The figure shows three views and two pictorial views of one solid part (mm, origin at its lowest corner). Answer the questions. Give positions to 0.01 mm unless a question says otherwise; leave off trailing zeros. Loops run counter-clockwise (first coordinate to the right, second up) from the corner with the lowest first, then second, coordinate; pieces in that order, holes last. Notation, with made-up numbers: (88, 69) - (128, 69) arc R22 cw to (128, 86) - close; hole circle Ø4 at (16.25, 87.5). An arc over 180 degrees is marked (long way). Write each question's results on one line, items separated by ' | '.
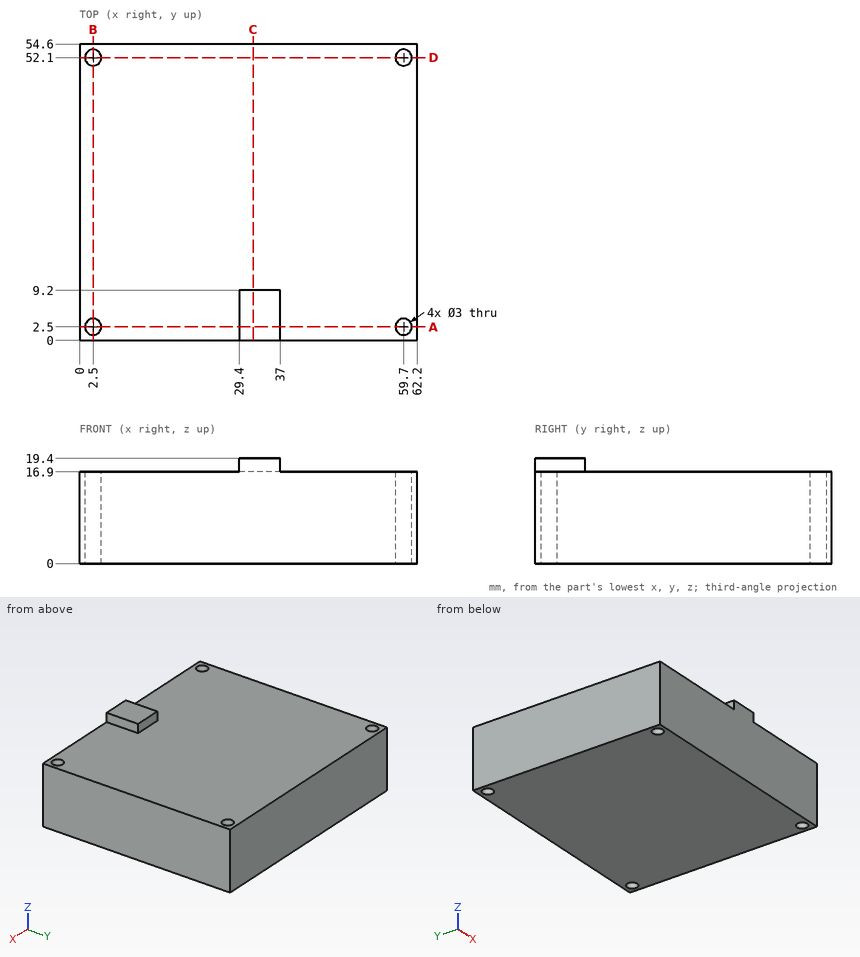
Item 1: A cutting plane is placed at C-C, the plane x = 32. Determine the outline of the cut face in (y, z), plus the area to 3 significant figures.
Values found:
outline: (0, 0) - (54.6, 0) - (54.6, 16.9) - (9.2, 16.9) - (9.2, 19.4) - (0, 19.4) - close | area: 946 mm²
Item 2: A cutting plane is placed at A-A, the plane y = 2.5. Determine the outline of the cut face in (x, z).
Values found:
outline: (0, 0) - (1, 0) - (1, 16.9) - (0, 16.9) - close; (4, 0) - (58.2, 0) - (58.2, 16.9) - (37, 16.9) - (37, 19.4) - (29.4, 19.4) - (29.4, 16.9) - (4, 16.9) - close; (61.2, 0) - (62.2, 0) - (62.2, 16.9) - (61.2, 16.9) - close
Item 3: A cutting plane is placed at B-B, the plane x = 2.5. Determine the outline of the cut face in (y, z).
Values found:
outline: (0, 0) - (1, 0) - (1, 16.9) - (0, 16.9) - close; (4, 0) - (50.6, 0) - (50.6, 16.9) - (4, 16.9) - close; (53.6, 0) - (54.6, 0) - (54.6, 16.9) - (53.6, 16.9) - close
Item 4: A cutting plane is placed at D-D, the plane y = 52.1. Determine the outline of the cut face in (x, z), plus the area to 3 significant figures.
Values found:
outline: (0, 0) - (1, 0) - (1, 16.9) - (0, 16.9) - close; (4, 0) - (58.2, 0) - (58.2, 16.9) - (4, 16.9) - close; (61.2, 0) - (62.2, 0) - (62.2, 16.9) - (61.2, 16.9) - close | area: 950 mm²
Item 5: Find the intervals of material crossed by line 1 along Y through (x, z) = (2.5, 11.25); line 2 along Z through (x, y) = (43, 32.5), in increasing order. Write a range as [from, to].
Values found:
line 1: y = [0, 1], [4, 50.6], [53.6, 54.6] | line 2: z = [0, 16.9]
Item 6: Flat-ended cylindrical pins translate along their axes: P1, Ø2, axis at x = 31.5, z = 18, coming from the +Y side; P2, Ø2.5, axis at x = 59.7, y = 52.1, coming from the -Z side; P3, Ø1.2, axis at y = 5, z = 18, coming from the -X side; P4, Ø1, axis at y = 6.5, z = 8, coming from the -X side. Find the tip coordinate at first contact, or state that the pin passes through.
Values found:
P1: stops at y = 9.2 | P2: passes through | P3: stops at x = 29.4 | P4: stops at x = 0
